Geometry check sheet. Reference: the model listing, model coordinates, mm. A direction names the side the tool comes from. Give positions to 0.01 mm unless a question says otherwise; leave off trailing zeros. Loops run counter-clockwise (first coordinate to the right, second up) from the corner with the lowest first, then second, coordinate; pieces in that order, holes last. Notation, with made-up numbers: (70, -28.5) -> (116, -28.5) arc R30 ccw to (116, 2.5) -> close; hole circle Ø10 at (55, 22). An arc over 180 degrees is marked (long way). Write item = value, one per line.
```python
from build123d import *

# Parameters (mm, degrees)
F0_W     = 10
F0_H     = 16
F1_DEPTH = 2
F3_DEPTH = 2


# Not quite as in the source:
# - ends of sketch curves that miss each other by under 0.0002 mm in the source are joined


with BuildPart() as f1:
    # F0 (on Top) → F1 (new body)
    with BuildSketch(Plane.XY):
        Rectangle(F0_W, F0_H)
    extrude(amount=F1_DEPTH)

    # F2 (on face) → F3 (join)
    with BuildSketch(Plane.XY.offset(2)):
        Polygon((0, 7), (-2, 7), (-3, 6), (-2, 5), (0, 5), (2, 5), (3, 6), (2, 7), align=None)
        Polygon((-2.1414213562, 4.8585786438), (-3.1414213562, 5.8585786438), (-4.1414213562, 4.8585786438), (-4.1414213562, 1.1507223826), (-3.1374518146, 0.1453992321), (-2.1414213562, 1.0335195075), align=None)
        Polygon((2, 0.891659756), (2.00782e-05, 0.9006214721), (-2, 0.891659756), (-3, 0), (-2, -0.891659756), (-2.00782e-05, -0.9006214721), (2, -0.891659756), (3, 0), align=None)
        Polygon((0, -5), (-2, -5), (-3, -6), (-2, -7), (0, -7), (2, -7), (3, -6), (2, -5), align=None)
        Polygon((-4.1414213562, -4.8585786438), (-3.1414213562, -5.8585786438), (-2.1414213562, -4.8585786438), (-2.1414213562, -1.0335195075), (-3.1374518146, -0.1453992321), (-4.1414213562, -1.1507223826), align=None)
        Polygon((4.1414213562, 4.8585786438), (3.1414213562, 5.8585786438), (2.1414213562, 4.8585786438), (2.1414213562, 1.0335195075), (3.1374518146, 0.1453992321), (4.1414213562, 1.1507223826), align=None)
        Polygon((3.1374518146, -0.1453992321), (2.1414213562, -1.0335195075), (2.1414213562, -4.8585786438), (3.1414213562, -5.8585786438), (4.1414213562, -4.8585786438), (4.1414213562, -1.1507223826), align=None)
    extrude(amount=F3_DEPTH)


solid = f1.part
```
Item 1: Gauge pin test, flat ends, axial feed: pin 1 (0.6 mm diameter, centred on x = 0.5, z = 3, fed in from -Y); pin 2 (1.6 mm diameter, centred on y = -3, z = 3, fed in from -X); pin 3 (1.6 mm diameter, centred on y = 3, z = 3, fed in from +X). Record the tip position at first contact, or that the pin passes through.
Answer:
pin_1 = -7
pin_2 = -4.14
pin_3 = 4.14
Item 2: Section check D-D, the plane x = -1. Record the cut outline in (y, z), plus the area to 3 significant figures.
Answer:
outline = (-8, 0) -> (8, 0) -> (8, 2) -> (7, 2) -> (7, 4) -> (5, 4) -> (5, 2) -> (0.9, 2) -> (0.9, 4) -> (-0.9, 4) -> (-0.9, 2) -> (-5, 2) -> (-5, 4) -> (-7, 4) -> (-7, 2) -> (-8, 2) -> close
area = 43.6 mm^2
Item 3: Section check C-C, the plane x = -2.5. Record the cut outline in (y, z).
Answer:
outline = (-8, 0) -> (8, 0) -> (8, 2) -> (6.5, 2) -> (6.5, 4) -> (5.5, 4) -> (5.5, 2) -> (5.22, 2) -> (5.22, 4) -> (0.71, 4) -> (0.71, 2) -> (0.45, 2) -> (0.45, 4) -> (-0.45, 4) -> (-0.45, 2) -> (-0.71, 2) -> (-0.71, 4) -> (-5.22, 4) -> (-5.22, 2) -> (-5.5, 2) -> (-5.5, 4) -> (-6.5, 4) -> (-6.5, 2) -> (-8, 2) -> close
Item 4: Draft check along Y on faces 6 (the flat face through (-2.634, 5.352, 2.986)), 7 (the flat face through (4, -5, 3)), 8 (the flat face through (3, -3, 4)). Enter one of: +Y half, -Y half, draft (parallel to the pull), parting line (faces both ways), or undercut.
Answer:
face_6 = undercut
face_7 = -Y half
face_8 = draft
Item 5: Tool access check on faces 1 (the flat face through (4.141, -3, 3)), 2 (the flat face through (-2.141, -3, 3)), 3 (the flat face through (0, -7, 3)), 4 (the flat face through (-4, -5, 3)), 5 (the flat face through (-3.65, 0.66, 2.99)). Record the directions out of +Z, -Z, +X, -X, +Y, -Y that give a thin tool (end or side, any length) a straight path to the whole face; none if there is none.
Answer:
face_1 = +Z, +X, +Y, -Y
face_2 = +Z
face_3 = +Z, +X, -X, -Y
face_4 = +Z, -X, -Y
face_5 = +Z, -X
Item 6: Section check B-B, the plane z = 3.05. Give the number of separate pieces and of enclosed holes in the cut face, plus the area to 3 significant figures.
Answer:
separate_pieces = 7
enclosed_holes = 0
area = 66.9 mm^2
Item 7: Section check A-A, the plane y = -3.25. Record the cut outline in (x, z), plus the area to 3 significant figures.
Answer:
outline = (-5, 0) -> (5, 0) -> (5, 2) -> (4.14, 2) -> (4.14, 4) -> (2.14, 4) -> (2.14, 2) -> (-2.14, 2) -> (-2.14, 4) -> (-4.14, 4) -> (-4.14, 2) -> (-5, 2) -> close
area = 28.0 mm^2
Item 8: Thickness scan on L1, parallel to Y at x = -1.25, z = 2.7; L2, parallel to Z at x = -1.5, y = 2; L3, parallel to X at y = 0.5, z = 2.4. Record the ranges inside material, lowest first. Write a range as [from, to].
Answer:
L1 = [-7, -5], [-0.9, 0.9], [5, 7]
L2 = [0, 2]
L3 = [-3.49, -2.74], [-2.44, 2.44], [2.74, 3.49]
